```python
from build123d import *

# Parameters (mm, degrees)
F1_DEPTH = 34.163


with BuildPart() as f1:
    # F0 (on Front) → F1 (new body, symmetric)
    with BuildSketch(Plane.XZ):
        with BuildLine():
            ThreePointArc((8.8900000424, 17.78), (2.6038207003, 2.6038207302), (17.78, 8.89))
            ThreePointArc((17.78, 8.89), (15.1761792997, 15.1761792698), (8.8900000424, 17.78))
        make_face()
        with BuildLine():
            ThreePointArc((26.67, 17.78), (20.3838207153, 15.1761792847), (17.78, 8.89))
            ThreePointArc((17.78, 8.89), (26.67, 0), (35.56, 8.89))
            ThreePointArc((35.56, 8.89), (32.9561792847, 15.1761792847), (26.67, 17.78))
        make_face()
        with BuildLine():
            ThreePointArc((8.8900000424, 17.78), (15.1761792997, 15.1761792698), (17.78, 8.89))
            ThreePointArc((17.78, 8.89), (20.3838207153, 15.1761792847), (26.67, 17.78))
            ThreePointArc((26.67, 17.78), (20.3838207153, 20.3838207153), (17.78, 26.67))
            ThreePointArc((17.78, 26.67), (15.1761792997, 20.3838207302), (8.8900000424, 17.78))
        make_face()
        with BuildLine():
            ThreePointArc((17.78, 26.67), (2.6038207003, 32.9561792698), (8.8900000424, 17.78))
            ThreePointArc((8.8900000424, 17.78), (15.1761792997, 20.3838207302), (17.78, 26.67))
        make_face()
        with BuildLine():
            ThreePointArc((44.45, 17.78), (38.1638207153, 15.1761792847), (35.56, 8.89))
            ThreePointArc((35.56, 8.89), (44.45, 0), (53.34, 8.89))
            ThreePointArc((53.34, 8.89), (50.7361792847, 15.1761792847), (44.45, 17.78))
        make_face()
        with BuildLine():
            ThreePointArc((26.67, 17.78), (32.9561792847, 15.1761792847), (35.56, 8.89))
            ThreePointArc((35.56, 8.89), (38.1638207153, 15.1761792847), (44.45, 17.78))
            ThreePointArc((44.45, 17.78), (38.1638207153, 20.3838207153), (35.56, 26.67))
            ThreePointArc((35.56, 26.67), (32.9561792847, 20.3838207153), (26.67, 17.78))
        make_face()
        with BuildLine():
            ThreePointArc((17.78, 26.67), (20.3838207153, 20.3838207153), (26.67, 17.78))
            ThreePointArc((26.67, 17.78), (32.9561792847, 20.3838207153), (35.56, 26.67))
            ThreePointArc((35.56, 26.67), (26.67, 35.56), (17.78, 26.67))
        make_face()
        with BuildLine():
            ThreePointArc((62.23, 17.78), (55.9438207153, 15.1761792847), (53.34, 8.89))
            ThreePointArc((53.34, 8.89), (62.23, 0), (71.12, 8.89))
            ThreePointArc((71.12, 8.89), (68.5161792847, 15.1761792847), (62.23, 17.78))
        make_face()
        with BuildLine():
            ThreePointArc((44.45, 17.78), (50.7361792847, 15.1761792847), (53.34, 8.89))
            ThreePointArc((53.34, 8.89), (55.9438207153, 15.1761792847), (62.23, 17.78))
            ThreePointArc((62.23, 17.78), (55.9438207153, 20.3838207153), (53.34, 26.67))
            ThreePointArc((53.34, 26.67), (50.7361792847, 20.3838207153), (44.45, 17.78))
        make_face()
        with BuildLine():
            ThreePointArc((35.56, 26.67), (38.1638207153, 20.3838207153), (44.45, 17.78))
            ThreePointArc((44.45, 17.78), (50.7361792847, 20.3838207153), (53.34, 26.67))
            ThreePointArc((53.34, 26.67), (44.45, 35.56), (35.56, 26.67))
        make_face()
        with BuildLine():
            ThreePointArc((80.01, 17.78), (73.7238207153, 15.1761792847), (71.12, 8.89))
            ThreePointArc((71.12, 8.89), (80.01, 0), (88.9, 8.89))
            ThreePointArc((88.9, 8.89), (86.2961792847, 15.1761792847), (80.01, 17.78))
        make_face()
        with BuildLine():
            ThreePointArc((62.23, 17.78), (68.5161792847, 15.1761792847), (71.12, 8.89))
            ThreePointArc((71.12, 8.89), (73.7238207153, 15.1761792847), (80.01, 17.78))
            ThreePointArc((80.01, 17.78), (73.7238207153, 20.3838207153), (71.12, 26.67))
            ThreePointArc((71.12, 26.67), (68.5161792847, 20.3838207153), (62.23, 17.78))
        make_face()
        with BuildLine():
            ThreePointArc((53.34, 26.67), (55.9438207153, 20.3838207153), (62.23, 17.78))
            ThreePointArc((62.23, 17.78), (68.5161792847, 20.3838207153), (71.12, 26.67))
            ThreePointArc((71.12, 26.67), (62.23, 35.56), (53.34, 26.67))
        make_face()
        with BuildLine():
            ThreePointArc((97.79, 17.78), (91.5038207153, 15.1761792847), (88.9, 8.89))
            ThreePointArc((88.9, 8.89), (97.79, 0), (106.68, 8.89))
            ThreePointArc((106.68, 8.89), (104.0761792847, 15.1761792847), (97.79, 17.78))
        make_face()
        with BuildLine():
            ThreePointArc((80.01, 17.78), (86.2961792847, 15.1761792847), (88.9, 8.89))
            ThreePointArc((88.9, 8.89), (91.5038207153, 15.1761792847), (97.79, 17.78))
            ThreePointArc((97.79, 17.78), (91.5038207153, 20.3838207153), (88.9, 26.67))
            ThreePointArc((88.9, 26.67), (86.2961792847, 20.3838207153), (80.01, 17.78))
        make_face()
        with BuildLine():
            ThreePointArc((71.12, 26.67), (73.7238207153, 20.3838207153), (80.01, 17.78))
            ThreePointArc((80.01, 17.78), (86.2961792847, 20.3838207153), (88.9, 26.67))
            ThreePointArc((88.9, 26.67), (80.01, 35.56), (71.12, 26.67))
        make_face()
        with BuildLine():
            ThreePointArc((115.57, 17.78), (109.2838207153, 15.1761792847), (106.68, 8.89))
            ThreePointArc((106.68, 8.89), (115.57, 0), (124.46, 8.89))
            ThreePointArc((124.46, 8.89), (121.8561792847, 15.1761792847), (115.57, 17.78))
        make_face()
        with BuildLine():
            ThreePointArc((97.79, 17.78), (104.0761792847, 15.1761792847), (106.68, 8.89))
            ThreePointArc((106.68, 8.89), (109.2838207153, 15.1761792847), (115.57, 17.78))
            ThreePointArc((115.57, 17.78), (109.2838207153, 20.3838207153), (106.68, 26.67))
            ThreePointArc((106.68, 26.67), (104.0761792847, 20.3838207153), (97.79, 17.78))
        make_face()
        with BuildLine():
            ThreePointArc((88.9, 26.67), (91.5038207153, 20.3838207153), (97.79, 17.78))
            ThreePointArc((97.79, 17.78), (104.0761792847, 20.3838207153), (106.68, 26.67))
            ThreePointArc((106.68, 26.67), (97.79, 35.56), (88.9, 26.67))
        make_face()
        with BuildLine():
            ThreePointArc((133.35, 17.78), (127.0638207153, 15.1761792847), (124.46, 8.89))
            ThreePointArc((124.46, 8.89), (133.35, 0), (142.24, 8.89))
            ThreePointArc((142.24, 8.89), (139.6361792847, 15.1761792847), (133.35, 17.78))
        make_face()
        with BuildLine():
            ThreePointArc((115.57, 17.78), (121.8561792847, 15.1761792847), (124.46, 8.89))
            ThreePointArc((124.46, 8.89), (127.0638207153, 15.1761792847), (133.35, 17.78))
            ThreePointArc((133.35, 17.78), (127.0638207153, 20.3838207153), (124.46, 26.67))
            ThreePointArc((124.46, 26.67), (121.8561792847, 20.3838207153), (115.57, 17.78))
        make_face()
        with BuildLine():
            ThreePointArc((106.68, 26.67), (109.2838207153, 20.3838207153), (115.57, 17.78))
            ThreePointArc((115.57, 17.78), (121.8561792847, 20.3838207153), (124.46, 26.67))
            ThreePointArc((124.46, 26.67), (115.57, 35.56), (106.68, 26.67))
        make_face()
        with BuildLine():
            ThreePointArc((124.46, 26.67), (127.0638207153, 20.3838207153), (133.35, 17.78))
            ThreePointArc((133.35, 17.78), (139.6361792847, 20.3838207153), (142.24, 26.67))
            ThreePointArc((142.24, 26.67), (133.35, 35.56), (124.46, 26.67))
        make_face()
    extrude(amount=F1_DEPTH, both=True)


solid = f1.part
```
Part model, mm, in its own coordinate system. Give positions to 0.01 mm unless a question says otherwise; leave off trailing zeros. Loops run counter-clockwise (first coordinate to the right, second up) from the corner with the lowest first, then second, coordinate; pieces in that order, holes last. Notation, with made-up numbers: M 7,58 L 47,58 A4 ccw 47,64 Z; hole C 70,40 d5. An arc over 180 degrees is marked long. Return JSON: item names as keys, results as strings.
1) Drill centre lines: line 1 (X direction, y = -14, z = 26); line 2 (Z direction, x = 26.5, y = 11.5); line 3 (Z direction, x = 98.5, y = 19). Where is each one in solid material? Low to high.
Calculated:
{"line 1": "x = 0.03 to 142.21", "line 2": "z = 0 to 35.56", "line 3": "z = 0.03 to 35.53"}
2) Saw through at A-A, the plane z = 31.5. Count the separate pieces of the cut face and the enclosed holes in it, then the cut area to 3 significant figures.
Calculated:
{"separate pieces": "8", "enclosed holes": "0", "area": "8,160 mm2"}
3) Flat gauge pins, fed straight in: pin 1 Ø6 at (y, z) = (-25.5, 21.5) entering from +X; pin 2 Ø5 at (y, z) = (-2.5, 16.5) entering from -X; pin 3 Ø8 at (y, z) = (22.5, 18.5) entering from -X. Where does each tip first touch, or does it go through?
Calculated:
{"pin 1": "stops at x = 141.97", "pin 2": "stops at x = 1.62", "pin 3": "stops at x = 1.04"}
4) Saw through at C-C, the plane x = 23. List the corners of the cut face in (y, z), then the cut area to 3 significant figures.
Calculated:
{"outline": "M -34.16,0.79 L 34.16,0.79 L 34.16,34.77 L -34.16,34.77 Z", "area": "2,320 mm2"}
5) Saw through at B-B, the plane y = -20. List the corners of the cut face in (x, z), then the cut area to 3 significant figures.
Calculated:
{"outline": "M 8.89,17.78 A8.89 ccw long 17.78,8.89 A8.89 ccw 35.56,8.89 A8.89 ccw 53.34,8.89 A8.89 ccw 71.12,8.89 A8.89 ccw 88.9,8.89 A8.89 ccw 106.68,8.89 A8.89 ccw 124.46,8.89 A8.89 ccw long 133.35,17.78 A8.89 ccw long 124.46,26.67 A8.89 ccw 106.68,26.67 A8.89 ccw 88.9,26.67 A8.89 ccw 71.12,26.67 A8.89 ccw 53.34,26.67 A8.89 ccw 35.56,26.67 A8.89 ccw 17.78,26.67 A8.89 ccw long Z", "area": "4,450 mm2"}
6) Pull direction Z, two halves, no side cores. Call faces 1 (the face through (70, -34.163, 18)), 2 (the face through (2.815, -0.478, 33.16)): released by +Z, released by -Z, zero draft, split by the parting line, or undercut.
Calculated:
{"face 1": "zero draft", "face 2": "undercut"}
